Input: part model. Units: mm. Frame: model coordinates. A direction names the side the tool comes from. Coordinates: 2 decimals unless noted, no trailing zeros. Order: outer loops, then holes, each group sorted by start corner. A loop starts at its lowest first (then second) coordinate and runs counter-clockwise, first axis right, second up. Notation, with made-up numbers: (82.25, -8) -> (141.25, -8) arc R4 cw to (141.25, -1) -> close; hole circle Ø1 at (-2.75, 6). An arc over 180 degrees is marked (long way). Answer as CSV lines item,"result".
Autodesk Inventor part; units mm, degrees
ref_plane "YZ Plane" through (0, 0, 0) normal (1, 0, 0) x (0, 1, 0)
ref_plane "XZ Plane" through (0, 0, 0) normal (0, 1, 0) x (-1, 0, 0)
ref_plane "XY Plane" through (0, 0, 0) normal (0, 0, 1) x (1, 0, 0)
sketch "스케치1" plane through (0, 0, 0) normal (0, 0, 1) x (1, 0, 0)
  line L0 (-50, -20) -> (50, -20)
  line L1 (50, 20) -> (-50, 20)
  line L2 (-50, -20) -> (50, 20) construction
  line L3 (50, -20) -> (-50, 20) construction
  arc A0 (-50, 20) -> (-50, -20) centre (-50, 0) ccw
  arc A1 (50, -20) -> (50, 20) centre (50, 0) ccw
  arc A2 (50, -30) -> (50, 30) centre (50, 0) ccw
  line L4 (50, -30) -> (-50, -30)
  arc A3 (-50, 30) -> (-50, -30) centre (-50, 0) ccw
  line L5 (25, 30) -> (25, 50)
  line L6 (-25, 30) -> (-25, 50)
  line L7 (-50, 30) -> (-25, 30)
  line L8 (25, 30) -> (50, 30)
  line L9 (-25, 50) -> (25, 50)
  point P0 (0, 0)
  point P1 (0, 0)
  dimension "d13" = 20
  dimension "d14" = 10
extrude "돌출1" add sketch "스케치1" along normal blind 50
sketch "스케치2" plane through (-25, 50, 0) normal (0, 1, 0) x (1, 0, 0)
  point P0 (25, 0)
ref_plane "작업 평면1" through (0, 0, 25) normal (0, 0, -1) x (-1, 0, 0)
sketch "스케치3" plane through (-25, 50, 0) normal (0, 1, 0) x (1, 0, 0)
  circle A0 centre (25, -25.091) radius 20
  point P0 (25, 0)
  dimension "d17" = 40
extrude "돌출2" add sketch "스케치3" along normal blind 100
sketch "스케치4" plane through (0, 0, 25) normal (0, 0, -1) x (-1, 0, 0)
  line L0 (50, -30) -> (-50, -30)
  line L1 (0, -30) -> (39.4468, -30)
  line L2 (39.4468, -30) -> (39.4468, -41.4109)
  line L3 (39.4468, -41.4109) -> (0, -41.4109)
  line L4 (0, -41.4109) -> (0, -30)
  point P0 (0, 0)
revolve "회전1" add sketch "스케치4" angle 360 about axis through (0, -41.4109, 25) along (0, 1, 0)
properties part number "부품1" material "은"
1. Cut plane A-A (y = 0). Return the cut outline in (x, z), plus the area to 3 significant figures.
Findings:
outline,"(-80, 0) -> (-70, 0) -> (-70, 50) -> (-80, 50) -> close; (70, 0) -> (80, 0) -> (80, 50) -> (70, 50) -> close"
area,"1,000 mm2"
2. Contact query for flat-ended pins moving along their axis: pin 1 (12 mm diameter, centred on y = 117, z = 12.5, fed in from -X); pin 2 (2 mm diameter, centred on x = -63.5, z = 45, fed in from +Y); pin 3 (10 mm diameter, centred on y = 40.5, z = 17, fed in from -X). Output: stop coordinate, or through.
Findings:
pin 1,"stops at x = -18.88"
pin 2,"stops at y = 27.27"
pin 3,"stops at x = -25"
3. Cut plane D-D (x = 0). Return the cut outline in (y, z).
Findings:
outline,"(-41.41, -14.45) -> (-30, -14.45) -> (-30, 0) -> (-20, 0) -> (-20, 50) -> (-30, 50) -> (-30, 64.45) -> (-41.41, 64.45) -> close; (20, 0) -> (50, 0) -> (50, 5.09) -> (150, 5.09) -> (150, 45.09) -> (50, 45.09) -> (50, 50) -> (20, 50) -> close"
4. Reachability of faces 4 (the face through (-17, 50, 14)), 5 (the face through (0, -30, 56)), 6 (the face through (25, 40, 25)) from +Z, -Z, +X, -X, +Y, -Y: full face, straight path, thin tool, end or side. Return the list, or none.
Findings:
face 4,"+Y"
face 5,"+Z, +X, -X, +Y"
face 6,"+Z, -Z, +X, +Y"
5. Cut plane C-C (z = 15). Return the cut outline in (x, y), plus the area to 3 significant figures.
Findings:
outline,"(-50, -30) -> (-38.16, -30) -> (-38.16, -41.41) -> (38.16, -41.41) -> (38.16, -30) -> (50, -30) arc R30 ccw to (50, 30) -> (25, 30) -> (25, 50) -> (17.27, 50) -> (17.27, 150) -> (-17.27, 150) -> (-17.27, 50) -> (-25, 50) -> (-25, 30) -> (-50, 30) arc R30 ccw to start; hole (-50, -20) -> (50, -20) arc R20 ccw to (50, 20) -> (-50, 20) arc R20 ccw to start"
area,"8,900 mm2"
6. Cut plane B-B (x = 47). Return the cut outline in (y, z), plus the area to 3 significant figures.
Findings:
outline,"(-30, 0) -> (-20, 0) -> (-20, 50) -> (-30, 50) -> close; (20, 0) -> (30, 0) -> (30, 50) -> (20, 50) -> close"
area,"1,000 mm2"
7. Mould query, pull axis Y, two halves, no side actions, for faces 1 (the face through (10.752, 99.3, 41.955)), 2 (the face through (-42, -30, 25)), 3 (the face through (-1, -20, 25)). Classes: released by +Y, released by -Y, zero draft, split by the parting line, or undercut.
Findings:
face 1,"zero draft"
face 2,"released by -Y"
face 3,"undercut"
8. Ray query, line 1 along Y through (x, z) = (-7.5, 2); line 2 along Y through (x, z) = (-46, 1); line 3 along Z through (x, y) = (-18, 26). Return the intervals inside material, ascending.
Findings:
line 1,"y = -41.41 to -20, 20 to 50"
line 2,"y = -30 to -20, 20 to 30"
line 3,"z = 0 to 50"
